```python
from build123d import *

# Parameters (mm, degrees)
F0_R     = 5.969
F0_R_2   = 4.8895
F1_DEPTH = 19.05


with BuildPart() as f1:
    # F0 (on Top) → F1 (new body)
    with BuildSketch(Plane.XY):
        Circle(F0_R)
        Circle(F0_R_2, mode=Mode.SUBTRACT)
    extrude(amount=-F1_DEPTH)


with BuildPart() as f2_1:
    # F2: copy of F1
    add(f1.part)


solid = f2_1.part
```
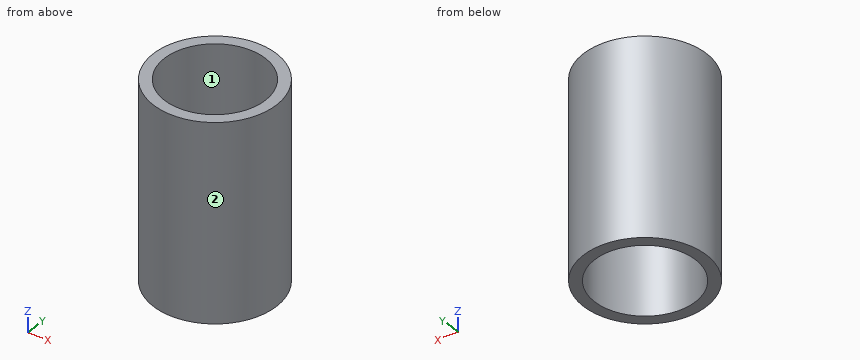
Read the model definition and answer for the solid it produces. Units are mm, in the model's axes. Face numbers are marked on the shaded views. Coordinates: 2 decimals unless noted, no trailing zeros. Write each loop counter-clockwise with the first axis right and the second up, starting at its lowest first coordinate (ties: lowest second). Pieces come first, ordered by that corner, then holes. Notation, with made-up numbers: (24.5, 27.5) - (37.5, 27.5) arc R20 ccw to (37.5, 62.5) - close; hole circle Ø1 at (60, 51). An arc over 180 degrees is marked (long way). Answer as a JSON object with one key per item and string values. Group by question number.
1. Consider L1, parallel to Y at x = 0, z = -7.5; L2, parallel to X at y = 1, z = -16.5. Determine where each line is inside the solid, lowest interval first. Write a range as [from, to].
2. A cutting plane is placed at B-B (y = 0.25). Determine the outline of the cut face in (x, z), plus the area to 3 significant figures.
3. A cutting plane is placed at A-A (x = 0). Determine the outline of the cut face in (y, z), plus the area to 3 significant figures.
4. The mould has two halves that part along X. Classify the marked faces 1 and 2: +X half, -X half, draft (parallel to the pull), parting line (faces both ways), or undercut.
5. A cutting plane is placed at C-C (z = -7.5). Determine the outline of the cut face in (x, y), plus the area to 3 significant figures.
Worked out:
{
 "1": {"L1": "y = [-5.97, -4.89], [4.89, 5.97]", "L2": "x = [-5.88, -4.79], [4.79, 5.88]"},
 "2": {"outline": "(-5.96, -19.05) - (-4.88, -19.05) - (-4.88, 0) - (-5.96, 0) - close; (4.88, -19.05) - (5.96, -19.05) - (5.96, 0) - (4.88, 0) - close", "area": "41.2 mm²"},
 "3": {"outline": "(-5.97, -19.05) - (-4.89, -19.05) - (-4.89, 0) - (-5.97, 0) - close; (4.89, -19.05) - (5.97, -19.05) - (5.97, 0) - (4.89, 0) - close", "area": "41.1 mm²"},
 "4": {"face 1": "undercut", "face 2": "parting line"},
 "5": {"outline": "circle Ø11.94 at (0, 0); hole circle Ø9.78 at (0, 0)", "area": "36.8 mm²"}
}
